Read the model definition and answer for the solid it produces. Units are mm, in the model's axes. Round coordinates to 2 decimals unless told otherwise and drop trailing zeros. Order: outer loops, then holes, each group sorted by start corner. A loop starts at its lowest first (then second) coordinate and runs counter-clockwise, first axis right, second up.
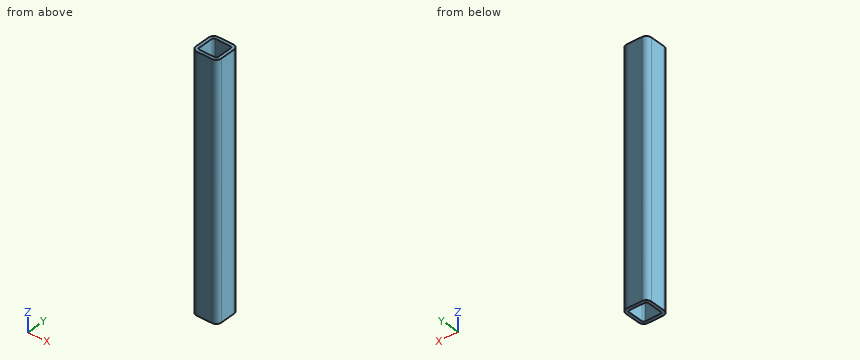
from build123d import *

# Parameters (mm, degrees)
SQUARE_TUBING_1_X_1_X_0_125_1_DEPTH = 251.1044


with BuildPart() as part:
    # Sketch11 → Square tubing 1 X 1 X 0.125(1) (new body)
    with BuildSketch(Plane.YX):
        with BuildLine():
            Line((-7.62, -12.7), (7.62, -12.7))
            ThreePointArc((7.62, -12.7), (11.212102448, -11.212102448), (12.7, -7.62))
            Line((12.7, -7.62), (12.7, 7.62))
            ThreePointArc((12.7, 7.62), (11.212102448, 11.212102448), (7.62, 12.7))
            Line((7.62, 12.7), (-7.62, 12.7))
            ThreePointArc((-7.62, 12.7), (-11.212102448, 11.212102448), (-12.7, 7.62))
            Line((-12.7, 7.62), (-12.7, -7.62))
            ThreePointArc((-12.7, -7.62), (-11.212102448, -11.212102448), (-7.62, -12.7))
        make_face()
        with BuildLine():
            Line((-7.62, -9.525), (7.62, -9.525))
            ThreePointArc((7.62, -9.525), (8.967038418, -8.967038418), (9.525, -7.62))
            Line((9.525, -7.62), (9.525, 7.62))
            ThreePointArc((9.525, 7.62), (8.967038418, 8.967038418), (7.62, 9.525))
            Line((7.62, 9.525), (-7.62, 9.525))
            ThreePointArc((-7.62, 9.525), (-8.967038418, 8.967038418), (-9.525, 7.62))
            Line((-9.525, 7.62), (-9.525, -7.62))
            ThreePointArc((-9.525, -7.62), (-8.967038418, -8.967038418), (-7.62, -9.525))
        make_face(mode=Mode.SUBTRACT)
    extrude(amount=SQUARE_TUBING_1_X_1_X_0_125_1_DEPTH)


solid = part.part
Q1. Straight lines are drawn through the part: probe 1 along Y at (x, z) = (1, -183.5) (3 decimals); probe 2 along Y at (x, z) = (-8.5, -64). For each, find the intervals that lie inside material, in ascending order.
Outcome:
probe 1: y = -12.7 to -9.525, 9.525 to 12.7
probe 2: y = -12.62 to -9.31, 9.31 to 12.62
Q2. A cutting plane is placed at C-C, the plane z = -174. Give the vertices of the cut face in (x, y) (3 decimals), plus the area to 3 significant figures.
Outcome:
outline: (-12.7, -7.62) arc R5.08 ccw to (-7.62, -12.7) - (7.62, -12.7) arc R5.08 ccw to (12.7, -7.62) - (12.7, 7.62) arc R5.08 ccw to (7.62, 12.7) - (-7.62, 12.7) arc R5.08 ccw to (-12.7, 7.62) - close; hole (-9.525, -7.62) arc R1.905 ccw to (-7.62, -9.525) - (7.62, -9.525) arc R1.905 ccw to (9.525, -7.62) - (9.525, 7.62) arc R1.905 ccw to (7.62, 9.525) - (-7.62, 9.525) arc R1.905 ccw to (-9.525, 7.62) - close
area: 263 mm2
Q3. A flat-ended cylindrical pin translates along its axis: pin 1 (10 mm diameter, centred on y = 8, z = -90, fed in from +X). Find the tip coordinate at first contact, or state that the pin passes through.
Outcome:
pin 1: stops at x = 12.7
Q4. A cutting plane is placed at A-A, the plane x = 0.25. Give the vertices of the cut face in (y, z) (3 decimals).
Outcome:
outline: (-12.7, -251.104) - (-9.525, -251.104) - (-9.525, 0) - (-12.7, 0) - close; (9.525, -251.104) - (12.7, -251.104) - (12.7, 0) - (9.525, 0) - close
